CAD build for the part. Positions are in the model's coordinates, mm. Coordinates: 2 decimals unless noted, no trailing zeros. Loops run counter-clockwise (first coordinate to the right, second up) from the corner with the lowest first, then second, coordinate; pieces in that order, holes last.
1) Saw through at B-B, the plane y = 0. Write the cut outline in (x, z).
2) Saw through at D-D, the plane y = -7. Write the cut outline in (x, z).
3) Two-plate mould, pull along X, no slides. Class faces 1 (the cylindrical face through (51.019, 17.647, -4.056)), 2 (the cylindrical face through (-43.661, 4.213, -3.944)), 3 (the flat face through (-1, 0, -8)): +X half, -X half, draft (parallel to the pull), parting line (faces both ways), or undercut.
4) Saw through at A-A, the plane x = 33.5. Write the cut outline in (y, z).
5) Wall check: line 1 along X through (y, z) = (0.5, -6.25); line 2 along Y through (x, z) = (-33.5, -4); line 3 along X through (y, z) = (-5, -7). Give the ranges that are in metal, low to high.
6) Saw through at C-C, the plane z = -3.75. Write the cut outline in (x, y).
Autodesk Inventor part; units mm, degrees
ref_plane "YZ Plane" through (0, 0, 0) normal (1, 0, 0) x (0, 1, 0)
ref_plane "XZ Plane" through (0, 0, 0) normal (0, 1, 0) x (-1, 0, 0)
ref_plane "XY Plane" through (0, 0, 0) normal (0, 0, 1) x (1, 0, 0)
sketch "Sketch1" plane through (0, 0, 0) normal (0, 0, 1) x (1, 0, 0)
  line L0 (-22.5, 0) -> (22.5, 0) construction
  circle A0 centre (33.5, 0) radius 11
  line L1 (-53.5, -20) -> (53.5, -20)
  line L2 (53.5, -20) -> (53.5, 20)
  line L3 (53.5, 20) -> (-53.5, 20)
  line L4 (-53.5, 20) -> (-53.5, -20)
  line L5 (-53.5, -20) -> (53.5, 20) construction
  line L6 (53.5, -20) -> (-53.5, 20) construction
  point P0 (0, 0)
  point P1 (0, 0)
  dimension "d4" = 22
  dimension "d3" = 45
  dimension "d11" = 20
  dimension "d12" = 20
extrude "Extrusion1" add sketch "Sketch1" against normal blind 8 contours A0 | L4 L3 L2 L1
extrude "Extrusion2" cut sketch "Sketch1" against normal through all contours A0
mirror "Mirror1" about plane through (0, 0, 0) normal (1, 0, 0) of "Extrusion2"
fillet "Fillet1" radius 8.25 4 edges at (-53.5, 20, -4) (53.5, 20, -4) (53.5, -20, -4) (-53.5, -20, -4)
properties part number "WeldAntiWarp"
Data:
1. outline: (-53.5, -8) - (-44.5, -8) - (-44.5, 0) - (-53.5, 0) - close; (-22.5, -8) - (22.5, -8) - (22.5, 0) - (-22.5, 0) - close; (44.5, -8) - (53.5, -8) - (53.5, 0) - (44.5, 0) - close
2. outline: (-53.5, -8) - (-41.99, -8) - (-41.99, 0) - (-53.5, 0) - close; (-25.01, -8) - (25.01, -8) - (25.01, 0) - (-25.01, 0) - close; (41.99, -8) - (53.5, -8) - (53.5, 0) - (41.99, 0) - close
3. face 1: +X half
3. face 2: undercut
3. face 3: draft
4. outline: (-20, -8) - (-11, -8) - (-11, 0) - (-20, 0) - close; (11, -8) - (20, -8) - (20, 0) - (11, 0) - close
5. line 1: x = -53.5 to -44.49, -22.51 to 22.51, 44.49 to 53.5
5. line 2: y = -20 to -11, 11 to 20
5. line 3: x = -53.5 to -43.3, -23.7 to 23.7, 43.3 to 53.5
6. outline: (-53.5, -11.75) arc R8.25 ccw to (-45.25, -20) - (45.25, -20) arc R8.25 ccw to (53.5, -11.75) - (53.5, 11.75) arc R8.25 ccw to (45.25, 20) - (-45.25, 20) arc R8.25 ccw to (-53.5, 11.75) - close; hole circle Ø22 at (-33.5, 0); hole circle Ø22 at (33.5, 0)
